The model under review builds one solid part; all positions refer to its coordinate system, in mm. Coordinates: 2 decimals unless noted, no trailing zeros. Order: outer loops, then holes, each group sorted by start corner. A loop starts at its lowest first (then second) coordinate and runs counter-clockwise, first axis right, second up. Notation, with made-up numbers: (-14, 35.5) -> (9, 35.5) arc R15 cw to (9, 43.5) -> close; hole circle Ø8 at (70, 88). An arc over 180 degrees is marked (long way). Use one line per item in the form item = value.
from build123d import *

# Parameters (mm, degrees)
SKETCH1_R           = 30
BOSS_EXTRUDE1_DEPTH = 7.5
CUT_EXTRUDE2_DEPTH  = 5.5
SKETCH6_R           = 6.25
CUT_EXTRUDE3_DEPTH  = 3
SKETCH9_R           = 1.5
BOSS_EXTRUDE5_DEPTH = 2
SKETCH10_R          = 2.5
BOSS_EXTRUDE6_DEPTH = 2


with BuildPart() as part:
    # Sketch1 → Boss-Extrude1 (new body)
    with BuildSketch(Plane(origin=(0, 0, 0), x_dir=(0, 0, -1), z_dir=(1, 0, 0))):
        Circle(SKETCH1_R)
    extrude(amount=BOSS_EXTRUDE1_DEPTH)

    # Sketch4 → Cut-Extrude2 (cut)
    with BuildSketch(Plane(origin=(7.5, 0, 0), x_dir=(0, -1, 0), z_dir=(1, 0, 0))):
        Polygon((8.200315972, -23.949003355), (8.095646912, -20.796423541), (10.150000757, -23.190028641), (9.785351218, -20.056859988), (12.030350745, -22.272642516), (11.408211652, -19.180287743), (13.828521239, -21.20311166), (12.953142433, -18.172694685), (15.532228911, -19.988742051), (14.409590118, -17.040963696), (17.12983571, -18.637829065), (15.76760569, -15.792825644), (18.610428362, -17.159600809), (17.017912527, -14.43680658), (19.963892917, -15.564155079), (18.151969766, -12.982169489), (21.18098384, -13.862390389), (19.162030646, -11.438851016), (22.253387167, -12.065931515), (20.041195426, -9.817393592), (23.173777294, -10.187050095), (20.78345852, -8.128873414), (23.935867025, -8.238580793), (21.383749518, -6.384824789), (24.534450513, -6.233833631), (21.837967824, -4.597161336), (24.965438827, -4.186503063), (22.143010666, -2.77809461), (25.225887879, -2.110574435), (22.296794293, -0.940050681), (25.314018538, -0.020228443), (22.298268206, 0.904414747), (25.229228782, 2.070255729), (22.147422337, 2.742702106), (24.972097812, 4.146597956), (21.845287117, 4.562254028), (24.544382092, 6.194614714), (21.393926434, 6.350641129), (23.949003355, 8.200315972), (20.796423541, 8.095646912), (23.190028641, 10.150000757), (20.056859988, 9.785351218), (22.272642516, 12.030350745), (19.180287743, 11.408211652), (21.20311166, 13.828521239), (18.172694685, 12.953142433), (19.988742051, 15.532228911), (17.040963696, 14.409590118), (18.637829065, 17.12983571), (15.792825644, 15.76760569), (17.159600809, 18.610428362), (14.43680658, 17.017912527), (15.564155079, 19.963892917), (12.982169489, 18.151969766), (13.862390389, 21.18098384), (11.438851016, 19.162030646), (12.065931515, 22.253387167), (9.817393592, 20.041195426), (10.187050095, 23.173777294), (8.128873414, 20.78345852), (8.238580793, 23.935867025), (6.384824789, 21.383749518), (6.233833631, 24.534450513), (4.597161336, 21.837967824), (4.186503063, 24.965438827), (2.77809461, 22.143010666), (2.110574435, 25.225887879), (0.940050681, 22.296794293), (0.020228443, 25.314018538), (-0.904414747, 22.298268206), (-2.070255729, 25.229228782), (-2.742702106, 22.147422337), (-4.146597956, 24.972097812), (-4.562254028, 21.845287117), (-6.194614714, 24.544382092), (-6.350641129, 21.393926434), (-8.200315972, 23.949003355), (-8.095646912, 20.796423541), (-10.150000757, 23.190028641), (-9.785351218, 20.056859988), (-12.030350745, 22.272642516), (-11.408211652, 19.180287743), (-13.828521239, 21.20311166), (-12.953142433, 18.172694685), (-15.532228911, 19.988742051), (-14.409590118, 17.040963696), (-17.12983571, 18.637829065), (-15.76760569, 15.792825644), (-18.610428362, 17.159600809), (-17.017912527, 14.43680658), (-19.963892917, 15.564155079), (-18.151969766, 12.982169489), (-21.18098384, 13.862390389), (-19.162030646, 11.438851016), (-22.253387167, 12.065931515), (-20.041195426, 9.817393592), (-23.173777294, 10.187050095), (-20.78345852, 8.128873414), (-23.935867025, 8.238580793), (-21.383749518, 6.384824789), (-24.534450513, 6.233833631), (-21.837967824, 4.597161336), (-24.965438827, 4.186503063), (-22.143010666, 2.77809461), (-25.225887879, 2.110574435), (-22.296794293, 0.940050681), (-25.314018538, 0.020228443), (-22.298268206, -0.904414747), (-25.229228782, -2.070255729), (-22.147422337, -2.742702106), (-24.972097812, -4.146597956), (-21.845287117, -4.562254028), (-24.544382092, -6.194614714), (-21.393926434, -6.350641129), (-23.949003355, -8.200315972), (-20.796423541, -8.095646912), (-23.190028641, -10.150000757), (-20.056859988, -9.785351218), (-22.272642516, -12.030350745), (-19.180287743, -11.408211652), (-21.20311166, -13.828521239), (-18.172694685, -12.953142433), (-19.988742051, -15.532228911), (-17.040963696, -14.409590118), (-18.637829065, -17.12983571), (-15.792825644, -15.76760569), (-17.159600809, -18.610428362), (-14.43680658, -17.017912527), (-15.564155079, -19.963892917), (-12.982169489, -18.151969766), (-13.862390389, -21.18098384), (-11.438851016, -19.162030646), (-12.065931515, -22.253387167), (-9.817393592, -20.041195426), (-10.187050095, -23.173777294), (-8.128873414, -20.78345852), (-8.238580793, -23.935867025), (-6.384824789, -21.383749518), (-6.233833631, -24.534450513), (-4.597161336, -21.837967824), (-4.186503063, -24.965438827), (-2.77809461, -22.143010666), (-2.110574435, -25.225887879), (-0.940050681, -22.296794293), (-0.020228443, -25.314018538), (0.904414747, -22.298268206), (2.070255729, -25.229228782), (2.742702106, -22.147422337), (4.146597956, -24.972097812), (4.562254028, -21.845287117), (6.194614714, -24.544382092), (6.350641129, -21.393926434), align=None)
    extrude(amount=-CUT_EXTRUDE2_DEPTH, mode=Mode.SUBTRACT)

    # Sketch6 → Cut-Extrude3 (cut, through all)
    with BuildSketch(Plane(origin=(2, 0, 0), x_dir=(0, 0, -1), z_dir=(1, 0, 0))):
        Circle(SKETCH6_R)
    extrude(amount=-CUT_EXTRUDE3_DEPTH, mode=Mode.SUBTRACT)

    # Sketch9 → Boss-Extrude5 (add)
    with BuildSketch(Plane(origin=(7.5, 0, 0), x_dir=(0, 0, -1), z_dir=(1, 0, 0))):
        with Locations((-19.065690414, 20.634386461)):
            Circle(SKETCH9_R)
    extrude(amount=BOSS_EXTRUDE5_DEPTH)

    # Sketch10 → Boss-Extrude6 (add)
    with BuildSketch(Plane(origin=(9.5, 0, 0), x_dir=(0, 0, -1), z_dir=(1, 0, 0))):
        with Locations((-19.065690414, 20.634386461)):
            Circle(SKETCH10_R)
    extrude(amount=BOSS_EXTRUDE6_DEPTH)


solid = part.part
Item 1: We need section A-A (y = -5.5). Write out the cut boundary in (x, z).
Results found:
outline = (0, -29.49) -> (7.5, -29.49) -> (7.5, -23.33) -> (2, -23.33) -> (2, -2.97) -> (0, -2.97) -> close; (0, 2.97) -> (2, 2.97) -> (2, 23.4) -> (7.5, 23.4) -> (7.5, 29.49) -> (0, 29.49) -> close
Item 2: Clearance check with flat-ended pins moving along their axes: pin 1 (1.5 mm diameter, centred on x = 9.5, z = -4, fed in from +Y); pin 2 (20 mm diameter, centred on y = 0, z = 0, fed in from +X); pin 3 (1.5 mm diameter, centred on x = 6.5, y = 19.5, fed in from +Z); pin 4 (6 mm diameter, centred on y = -22.5, z = -21.5, fed in from +X). State where each tip first meets the part, or that it passes through.
Results found:
pin_1 = through
pin_2 = 2
pin_3 = 23.42
pin_4 = 7.5
Item 3: To check wall thickness, follow L1, parallel to Y at x = 1.2, z = 0; L2, parallel to Z at x = 5.25, y = 12.5; L3, parallel to X at y = -4, z = 13. State the ranges of each line that lie inside material, in increasing order. Write a range as from..to.
Results found:
L1 = -30..-6.25, 6.25..30
L2 = -27.27..-20.09, 20.05..27.27
L3 = 0..2
Item 4: We need section B-B (x = 10.5). Write out the cut boundary in (y, z), plus the area to 3 significant figures.
Results found:
outline = circle Ø5 at (20.63, 19.07)
area = 19.6 mm²
Item 5: Draft analysis for pull direction Z (two halves, no side actions). For faces 1 (the face through (4.788, 16.467, 17.169)), 2 (the face through (10.486, 20.744, 21.563)), state which applies: released by +Z, released by -Z, zero draft, split by the parting line, or undercut.
Results found:
face_1 = undercut
face_2 = split by the parting line
